from build123d import *

# Parameters (mm, degrees)
SALIENTE_EXTRUIR1_DEPTH = 8


with BuildPart() as part:
    # Croquis1 → Saliente-Extruir1 (new body)
    with BuildSketch(Plane(origin=(0, 0, 0), x_dir=(1, 0, 0), z_dir=(0, 1, 0))):
        Polygon((12.124151894, 0.070291154), (6.001202022, 10.534969117), (-6.122949872, 10.464677963), (-12.124151894, -0.070291154), (-6.001202022, -10.534969117), (6.122949872, -10.464677963), align=None)
        Polygon((3.79039754, -6.478133977), (7.505427363, 0.043513571), (3.715029823, 6.521647548), (-3.79039754, 6.478133977), (-7.505427363, -0.043513571), (-3.715029823, -6.521647548), align=None, mode=Mode.SUBTRACT)
    extrude(amount=SALIENTE_EXTRUIR1_DEPTH)


solid = part.part
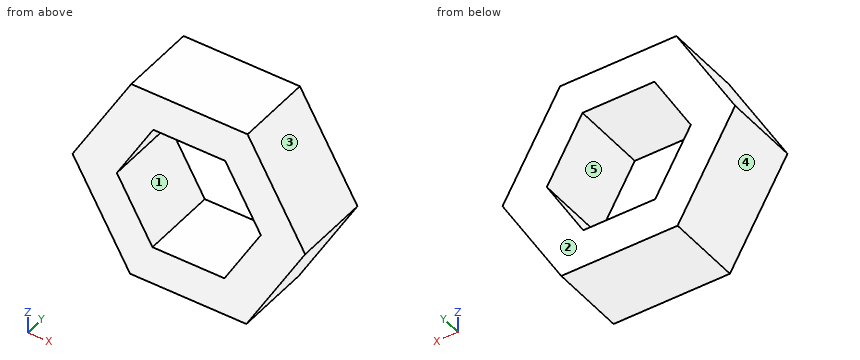
Design review of the part built by this model. Coordinates are the model's own, in mm. Face numbers are marked on the shaded views. A direction names the side the tool comes from. Give positions to 0.01 mm unless a question says otherwise; leave off trailing zeros. Write each loop counter-clockwise with the first axis right and the second up, starting at its lowest first coordinate (ties: lowest second). Pieces come first, ordered by that corner, then holes. Notation, with made-up numbers: M 28,42.5 L 69,42.5 A29 cw 69,76.5 Z; hole C 19.25,78 d5. An arc over 180 degrees is marked long. Answer as a JSON object with one key per item and string values. Group by question number.
1) We need section C-C (x = 0.25). Give the boundary of the cut face in (y, z).
2) We need section D-D (x = 10.25). Give the boundary of the cut face in (y, z).
3) Tool access review of the marked faces 4 and 5: name each direction out of +Z, -Z, +X, -X, +Y, -Y from which nothing blocks a thin tool from reaching the whole face with its end or side.
4) We need section B-B (z = -3). Give the boundary of the cut face in (x, y).
5) Mouldability with a two-part tool opening along X and no side actions: class the marked faces 1, 2 and 3 as released by +X, released by -X, zero draft, split by the parting line, or undercut.
6) We need section A-A (y = 5.5). Give the boundary of the cut face in (x, z).
7) Clearance check with flat-ended pins moving along their axes: pin 1 Ø2 at (y, z) = (7, -7.5) entering from +X; pin 2 Ø4 at (y, z) = (5, 8) entering from -X; pin 3 Ø1 at (y, z) = (7, 4) entering from -X. State where each tip first meets the part, or that it passes through.
8) For line 1 along X through (y, z) = (7.75, 0.75); line 2 along Z through (x, y) = (-6.5, 1.5); line 3 along Z through (x, y) = (2.5, 6), list the stretches that pass through material, from the lowest coordinate up.
Answer key:
{
 "1": {"outline": "M 0,-10.5 L 8,-10.5 L 8,-6.5 L 0,-6.5 Z; M 0,6.5 L 8,6.5 L 8,10.5 L 0,10.5 Z"},
 "2": {"outline": "M 0,-3.27 L 8,-3.27 L 8,3.22 L 0,3.22 Z"},
 "3": {"face 4": "-Z, -X, +Y, -Y", "face 5": "+Y, -Y"},
 "4": {"outline": "M -10.38,0 L -5.77,0 L -5.77,8 L -10.38,8 Z; M 5.78,0 L 10.41,0 L 10.41,8 L 5.78,8 Z"},
 "5": {"face 1": "undercut", "face 2": "zero draft", "face 3": "released by +X"},
 "6": {"outline": "M -12.12,0.07 L -6.12,-10.46 L 6,-10.53 L 12.12,-0.07 L 6.12,10.46 L -6,10.53 Z; hole M -7.51,0.04 L -3.79,-6.48 L 3.72,-6.52 L 7.51,-0.04 L 3.79,6.48 L -3.72,6.52 Z"},
 "7": {"pin 1": "stops at x = 8.36", "pin 2": "stops at x = -8.65", "pin 3": "stops at x = -10.12"},
 "8": {"line 1": "x = -11.73 to -7.09, 7.05 to 11.66", "line 2": "z = -9.8 to -1.72, 1.76 to 9.68", "line 3": "z = -10.51 to -6.51, 6.49 to 10.49"}
}
